```python
from build123d import *

# Parameters (mm, degrees)
BOSS_EXTRUDE1_DEPTH = 4
SKETCH2_W           = 4
SKETCH2_H           = 4
CUT_EXTRUDE1_DEPTH  = 3
FILLET1_R           = 0.25


with BuildPart() as part:
    # Sketch1 → Boss-Extrude1 (new body)
    with BuildSketch(Plane(origin=(0, 0, 0), x_dir=(1, 0, 0), z_dir=(0, 1, 0))):
        Polygon((3.214834695, -1.383776673), (2.8058031, 2.092240179), (-0.409031596, 3.476016852), (-3.214834695, 1.383776673), (-2.8058031, -2.092240179), (0.409031596, -3.476016852), align=None)
    extrude(amount=BOSS_EXTRUDE1_DEPTH)

    # Sketch2 → Cut-Extrude1 (cut)
    with BuildSketch(Plane(origin=(0, 4, 0), x_dir=(1, 0, 0), z_dir=(0, 1, 0))):
        Rectangle(SKETCH2_W, SKETCH2_H)
    extrude(amount=-CUT_EXTRUDE1_DEPTH, mode=Mode.SUBTRACT)

    # Fillet1
    # the kernel refuses this fillet: 0.25 mm, written as the material it takes off along each edge
    with BuildSketch(Plane(origin=(-2, 4, -2), x_dir=(-1, 0, 0), z_dir=(0, 0, 1)), Plane(origin=(2, 4, -2), x_dir=(0, 0, -1), z_dir=(-1, 0, 0)), Plane(origin=(-2, 4, 2), x_dir=(0, 0, 1), z_dir=(1, 0, 0)), Plane(origin=(2, 4, 2), x_dir=(1, 0, 0), z_dir=(0, 0, -1))) as fillet1_piece_1:
        with BuildLine():
            CenterArc((FILLET1_R, FILLET1_R), FILLET1_R, 180, 90)
            Line((0, FILLET1_R), (-FILLET1_R * 0.02, FILLET1_R))
            Line((-FILLET1_R * 0.02, FILLET1_R), (-FILLET1_R * 0.02, -FILLET1_R * 0.02))
            Line((-FILLET1_R * 0.02, -FILLET1_R * 0.02), (FILLET1_R, -FILLET1_R * 0.02))
            Line((FILLET1_R, -FILLET1_R * 0.02), (FILLET1_R, 0))
        make_face()
    extrude(amount=4, mode=Mode.SUBTRACT)
    with BuildSketch(Plane(origin=(2, 4, -2), x_dir=(0, 0, -1), z_dir=(-1, 0, 0))) as fillet1_piece_2a_section:
        with BuildLine():
            CenterArc((FILLET1_R, FILLET1_R), FILLET1_R, 180, 90)
            Line((0, FILLET1_R), (-FILLET1_R * 0.02, FILLET1_R))
            Line((-FILLET1_R * 0.02, FILLET1_R), (-FILLET1_R * 0.02, -FILLET1_R * 0.02))
            Line((-FILLET1_R * 0.02, -FILLET1_R * 0.02), (FILLET1_R, -FILLET1_R * 0.02))
            Line((FILLET1_R, -FILLET1_R * 0.02), (FILLET1_R, 0))
        make_face()
    fillet1_piece_2a = extrude(amount=4.625, mode=Mode.PRIVATE)
    fillet1_piece_2a = split(fillet1_piece_2a, bisect_by=Plane(origin=(-2, 3.943401221, -2.056598779), z_dir=(-1, 0, 0)), keep=Keep.TOP, mode=Mode.PRIVATE)
    with BuildSketch(Plane(origin=(-2, 4, -2.625), x_dir=(-1, 0, 0), z_dir=(0, 0, 1))) as fillet1_piece_2b_section:
        with BuildLine():
            CenterArc((FILLET1_R, FILLET1_R), FILLET1_R, 180, 90)
            Line((0, FILLET1_R), (-FILLET1_R * 0.02, FILLET1_R))
            Line((-FILLET1_R * 0.02, FILLET1_R), (-FILLET1_R * 0.02, -FILLET1_R * 0.02))
            Line((-FILLET1_R * 0.02, -FILLET1_R * 0.02), (FILLET1_R, -FILLET1_R * 0.02))
            Line((FILLET1_R, -FILLET1_R * 0.02), (FILLET1_R, 0))
        make_face()
    fillet1_piece_2b = extrude(amount=4.625, mode=Mode.PRIVATE)
    fillet1_piece_2b = split(fillet1_piece_2b, bisect_by=Plane(origin=(-2.056598779, 3.943401221, -2), z_dir=(0, 0, -1)), keep=Keep.TOP, mode=Mode.PRIVATE)
    fillet1_piece_2 = fillet1_piece_2a & fillet1_piece_2b
    add(fillet1_piece_2, mode=Mode.SUBTRACT)
    with BuildSketch(Plane(origin=(-2.625, 4, 2), x_dir=(0, 0, 1), z_dir=(1, 0, 0))) as fillet1_piece_3a_section:
        with BuildLine():
            CenterArc((FILLET1_R, FILLET1_R), FILLET1_R, 180, 90)
            Line((0, FILLET1_R), (-FILLET1_R * 0.02, FILLET1_R))
            Line((-FILLET1_R * 0.02, FILLET1_R), (-FILLET1_R * 0.02, -FILLET1_R * 0.02))
            Line((-FILLET1_R * 0.02, -FILLET1_R * 0.02), (FILLET1_R, -FILLET1_R * 0.02))
            Line((FILLET1_R, -FILLET1_R * 0.02), (FILLET1_R, 0))
        make_face()
    fillet1_piece_3a = extrude(amount=4.625, mode=Mode.PRIVATE)
    fillet1_piece_3a = split(fillet1_piece_3a, bisect_by=Plane(origin=(-2, 3.943401221, 2.056598779), z_dir=(-1, 0, 0)), keep=Keep.TOP, mode=Mode.PRIVATE)
    with BuildSketch(Plane(origin=(-2, 4, -2), x_dir=(-1, 0, 0), z_dir=(0, 0, 1))) as fillet1_piece_3b_section:
        with BuildLine():
            CenterArc((FILLET1_R, FILLET1_R), FILLET1_R, 180, 90)
            Line((0, FILLET1_R), (-FILLET1_R * 0.02, FILLET1_R))
            Line((-FILLET1_R * 0.02, FILLET1_R), (-FILLET1_R * 0.02, -FILLET1_R * 0.02))
            Line((-FILLET1_R * 0.02, -FILLET1_R * 0.02), (FILLET1_R, -FILLET1_R * 0.02))
            Line((FILLET1_R, -FILLET1_R * 0.02), (FILLET1_R, 0))
        make_face()
    fillet1_piece_3b = extrude(amount=4.625, mode=Mode.PRIVATE)
    fillet1_piece_3b = split(fillet1_piece_3b, bisect_by=Plane(origin=(-2.056598779, 3.943401221, 2), z_dir=(0, 0, 1)), keep=Keep.TOP, mode=Mode.PRIVATE)
    fillet1_piece_3 = fillet1_piece_3a & fillet1_piece_3b
    add(fillet1_piece_3, mode=Mode.SUBTRACT)
    with BuildSketch(Plane(origin=(2, 4, 2), x_dir=(1, 0, 0), z_dir=(0, 0, -1))) as fillet1_piece_4a_section:
        with BuildLine():
            CenterArc((FILLET1_R, FILLET1_R), FILLET1_R, 180, 90)
            Line((0, FILLET1_R), (-FILLET1_R * 0.02, FILLET1_R))
            Line((-FILLET1_R * 0.02, FILLET1_R), (-FILLET1_R * 0.02, -FILLET1_R * 0.02))
            Line((-FILLET1_R * 0.02, -FILLET1_R * 0.02), (FILLET1_R, -FILLET1_R * 0.02))
            Line((FILLET1_R, -FILLET1_R * 0.02), (FILLET1_R, 0))
        make_face()
    fillet1_piece_4a = extrude(amount=4.625, mode=Mode.PRIVATE)
    fillet1_piece_4a = split(fillet1_piece_4a, bisect_by=Plane(origin=(2.056598779, 3.943401221, -2), z_dir=(0, 0, -1)), keep=Keep.TOP, mode=Mode.PRIVATE)
    with BuildSketch(Plane(origin=(2.625, 4, -2), x_dir=(0, 0, -1), z_dir=(-1, 0, 0))) as fillet1_piece_4b_section:
        with BuildLine():
            CenterArc((FILLET1_R, FILLET1_R), FILLET1_R, 180, 90)
            Line((0, FILLET1_R), (-FILLET1_R * 0.02, FILLET1_R))
            Line((-FILLET1_R * 0.02, FILLET1_R), (-FILLET1_R * 0.02, -FILLET1_R * 0.02))
            Line((-FILLET1_R * 0.02, -FILLET1_R * 0.02), (FILLET1_R, -FILLET1_R * 0.02))
            Line((FILLET1_R, -FILLET1_R * 0.02), (FILLET1_R, 0))
        make_face()
    fillet1_piece_4b = extrude(amount=4.625, mode=Mode.PRIVATE)
    fillet1_piece_4b = split(fillet1_piece_4b, bisect_by=Plane(origin=(2, 3.943401221, -2.056598779), z_dir=(1, 0, 0)), keep=Keep.TOP, mode=Mode.PRIVATE)
    fillet1_piece_4 = fillet1_piece_4a & fillet1_piece_4b
    add(fillet1_piece_4, mode=Mode.SUBTRACT)
    with BuildSketch(Plane(origin=(-2, 4, 2), x_dir=(0, 0, 1), z_dir=(1, 0, 0))) as fillet1_piece_5a_section:
        with BuildLine():
            CenterArc((FILLET1_R, FILLET1_R), FILLET1_R, 180, 90)
            Line((0, FILLET1_R), (-FILLET1_R * 0.02, FILLET1_R))
            Line((-FILLET1_R * 0.02, FILLET1_R), (-FILLET1_R * 0.02, -FILLET1_R * 0.02))
            Line((-FILLET1_R * 0.02, -FILLET1_R * 0.02), (FILLET1_R, -FILLET1_R * 0.02))
            Line((FILLET1_R, -FILLET1_R * 0.02), (FILLET1_R, 0))
        make_face()
    fillet1_piece_5a = extrude(amount=4.625, mode=Mode.PRIVATE)
    fillet1_piece_5a = split(fillet1_piece_5a, bisect_by=Plane(origin=(2, 3.943401221, 2.056598779), z_dir=(1, 0, 0)), keep=Keep.TOP, mode=Mode.PRIVATE)
    with BuildSketch(Plane(origin=(2, 4, 2.625), x_dir=(1, 0, 0), z_dir=(0, 0, -1))) as fillet1_piece_5b_section:
        with BuildLine():
            CenterArc((FILLET1_R, FILLET1_R), FILLET1_R, 180, 90)
            Line((0, FILLET1_R), (-FILLET1_R * 0.02, FILLET1_R))
            Line((-FILLET1_R * 0.02, FILLET1_R), (-FILLET1_R * 0.02, -FILLET1_R * 0.02))
            Line((-FILLET1_R * 0.02, -FILLET1_R * 0.02), (FILLET1_R, -FILLET1_R * 0.02))
            Line((FILLET1_R, -FILLET1_R * 0.02), (FILLET1_R, 0))
        make_face()
    fillet1_piece_5b = extrude(amount=4.625, mode=Mode.PRIVATE)
    fillet1_piece_5b = split(fillet1_piece_5b, bisect_by=Plane(origin=(2.056598779, 3.943401221, 2), z_dir=(0, 0, 1)), keep=Keep.TOP, mode=Mode.PRIVATE)
    fillet1_piece_5 = fillet1_piece_5a & fillet1_piece_5b
    add(fillet1_piece_5, mode=Mode.SUBTRACT)


solid = part.part
```
CAD build for the part. Positions are in the model's coordinates, mm. A direction names the side the tool comes from. Round coordinates to 2 decimals unless told otherwise and drop trailing zeros. Write each loop counter-clockwise with the first axis right and the second up, starting at its lowest first coordinate (ties: lowest second). Pieces come first, ordered by that corner, then holes. Notation, with made-up numbers: (18, -31.5) - (29, -31.5) arc R16 cw to (29, -8.5) - close; hole circle Ø4 at (28.5, 70). An arc over 180 degrees is marked (long way). Return JSON: item names as keys, results as strings. Group by question number.
Item 1: Flat gauge pins, fed straight in: pin 1 Ø2 at (y, z) = (2, 1) entering from -X; pin 2 Ø2 at (x, z) = (0, 0.5) entering from +Y; pin 3 Ø1 at (x, y) = (-0.5, 2.5) entering from -Z; pin 4 Ø1 at (x, y) = (2, 2.5) entering from +Z. Where does each tip first touch, or does it go through?
Item 2: Mould opens along X. For faces 1 (the face through (1.221, 1.972, -2.774)), 2 (the face through (-3.013, 1.972, 0.33)), 3 (the face through (0, 2, 2)), 4 (the face through (0, 2, -2)) say: +X half, -X half, draft (parallel to the pull), parting line (faces both ways), or undercut.
Item 3: 3-axis set-ups, long thin cutter, end or side, ignore diameter. For faces 5 (the face through (-2, 2, 0)), 6 (the face through (3.013, 1.972, -0.33)): which of +Z, -Z, +X, -X, +Y, -Y reach the whole face in a straight line?
Item 4: Probe probe 1 along Y at (x, z) = (1.75, 1.5); probe 2 along Z at (x, y) = (-0.75, 3.35); probe 3 along Z at (x, y) = (-1.25, 3.8). List the from-to ranges inside material, lowest first.
Item 5: Band-saw the part on D-D on x = 1.5. List the corners of the cut face in (y, z).
Item 6: Band-saw the part on B-B on z = -1.5. List the corners of the cut face in (x, y), plus the area to 3 significant figures.
Item 7: Band-saw the part on A-A on y = 2.65. List the corners of the cut face in (x, z), plus the area to 3 significant figures.
Item 8: Band-saw the part on C-C on y = 0.35. List the corners of the cut face in (x, z).
Resolved:
{
 "1": {"pin 1": "stops at x = -3.05", "pin 2": "stops at y = 1", "pin 3": "stops at z = -3.48", "pin 4": "stops at z = 2.66"},
 "2": {"face 1": "+X half", "face 2": "-X half", "face 3": "undercut", "face 4": "undercut"},
 "3": {"face 5": "+Y", "face 6": "-Z, +X, +Y, -Y"},
 "4": {"probe 1": "y = 0 to 1", "probe 2": "z = -3.22 to -2, 2 to 2.98", "probe 3": "z = -2.85 to -2.01, 2.01 to 2.76"},
 "5": {"outline": "(0, -2.65) - (4, -2.65) - (4, -2.25) arc R0.25 ccw to (3.75, -2) - (1, -2) - (1, 2) - (3.75, 2) arc R0.25 ccw to (4, 2.25) - (4, 2.66) - (0, 2.66) - close"},
 "6": {"outline": "(-3.06, 0) - (2.88, 0) - (2.88, 4) - (2.25, 4) arc R0.25 ccw to (2, 3.75) - (2, 1) - (-2, 1) - (-2, 3.75) arc R0.25 ccw to (-2.25, 4) - (-3.06, 4) - close", "area": "11.7 mm²"},
 "7": {"outline": "(-3.21, -1.38) - (-0.41, -3.48) - (2.81, -2.09) - (3.21, 1.38) - (0.41, 3.48) - (-2.81, 2.09) - close; hole (-2, -2) - (2, -2) - (2, 2) - (-2, 2) - close", "area": "15.8 mm²"},
 "8": {"outline": "(-3.21, -1.38) - (-0.41, -3.48) - (2.81, -2.09) - (3.21, 1.38) - (0.41, 3.48) - (-2.81, 2.09) - close"}
}
